Read the model definition and answer for the solid it produces. Units are mm, in the model's axes. A direction names the side the tool comes from. Coordinates: 2 decimals unless noted, no trailing zeros. Order: outer loops, then holes, each group sorted by start corner. A loop starts at its lowest first (then second) coordinate and runs counter-clockwise, first axis right, second up. Notation, with made-up numbers: (43, 0) - (101, 0) arc R16 cw to (101, 28) - close; hole circle Ø6 at (-32.5, 65). An arc over 180 degrees is marked (long way). Use one line per item in the form item = value.
```python
from build123d import *

# Parameters (mm, degrees)
F1_DEPTH = 0.5
F2_R     = 2.047791
F3_DEPTH = 9.5


with BuildPart() as f1:
    # F0 (on Top) → F1 (new body)
    with BuildSketch(Plane.XY):
        Polygon((16.35, 29.214), (-16.35, 29.214), (-16.35, 23.9715), (-9.35, 23.9715), (-9.35, 10.9715), (-16.35, 10.9715), (-16.35, 0), (-16.35, -10.9715), (-9.35, -10.9715), (-9.35, -23.9715), (-16.35, -23.9715), (-16.35, -29.214), (16.35, -29.214), (16.35, -23.9715), (9.35, -23.9715), (9.35, -10.9715), (16.35, -10.9715), (16.35, 0), (16.35, 10.9715), (9.35, 10.9715), (9.35, 23.9715), (16.35, 23.9715), align=None)
    extrude(amount=F1_DEPTH)

    # F2 (on Right) → F3 (join, symmetric)
    with BuildSketch(Plane.YZ):
        with BuildLine():
            Line((23.961247, 0), (10.961247, 0))
            ThreePointArc((10.961247, 0), (17.461247, -5.333223), (23.961247, 0))
        make_face()
        with Locations((17.461247, -2.643129)):
            Circle(F2_R, mode=Mode.SUBTRACT)
        with BuildLine():
            ThreePointArc((-23.961247, 0), (-17.461247, -5.333223), (-10.961247, 0))
            Line((-10.961247, 0), (-23.961247, 0))
        make_face()
        with Locations((-17.461247, -2.643129)):
            Circle(F2_R, mode=Mode.SUBTRACT)
    extrude(amount=F3_DEPTH, both=True)


solid = f1.part
```
(1) Which of the six approach directions +Z, -Z, +X, -X, +Y, -Y give full straight-line access (tool end or side, diameter ignored) to faces 3 (the flat face through (0, 27, 0)), 4 (the flat face through (0, 0, 0)), 5 (the cylindrical face through (-0.133, 15.836, -3.889)), 6 (the flat face through (0, -27, 0))?
Answer list:
face_3 = -Z, +X, -X, +Y
face_4 = -Z, +X, -X
face_5 = +X, -X
face_6 = -Z, +X, -X, -Y
(2) Straight lines are drawn through the part: L1, parallel to Y at x = 1, z = -0.05; L2, parallel to Y at x = -4.5, z = -1.05; L3, parallel to Y at x = -9, z = -3.2. For each, find the intervals that lie inside material, in ascending order.
Answer list:
L1 = -23.95 to -10.97, 10.97 to 23.95
L2 = -23.66 to -18.75, -16.17 to -11.26, 11.26 to 16.17, 18.75 to 23.66
L3 = -22.33 to -19.43, -15.49 to -12.59, 12.59 to 15.49, 19.43 to 22.33
(3) Section B-B, the plane z = -3.85 is taken. Write down the section's boundary in (x, y).
Answer list:
outline = (-9.5, -21.64) - (9.5, -21.64) - (9.5, -19.12) - (-9.5, -19.12) - close; (-9.5, -15.81) - (9.5, -15.81) - (9.5, -13.28) - (-9.5, -13.28) - close; (-9.5, 13.28) - (9.5, 13.28) - (9.5, 15.81) - (-9.5, 15.81) - close; (-9.5, 19.12) - (9.5, 19.12) - (9.5, 21.64) - (-9.5, 21.64) - close
(4) Section A-A, the plane x = -14 is taken. Write down the section's boundary in (y, z), then the cut area to 3 significant figures.
Answer list:
outline = (-29.21, 0) - (-23.97, 0) - (-23.97, 0.5) - (-29.21, 0.5) - close; (-10.97, 0) - (10.97, 0) - (10.97, 0.5) - (-10.97, 0.5) - close; (23.97, 0) - (29.21, 0) - (29.21, 0.5) - (23.97, 0.5) - close
area = 16.2 mm2
(5) Section C-C, the plane y = -18.5 is taken. Write down the section's boundary in (x, z), then the cut area to 3 significant figures.
Answer list:
outline = (-9.5, -5.25) - (9.5, -5.25) - (9.5, -4.41) - (-9.5, -4.41) - close; (-9.5, -0.88) - (9.5, -0.88) - (9.5, 0) - (9.35, 0) - (9.35, 0.5) - (-9.35, 0.5) - (-9.35, 0) - (-9.5, 0) - close
area = 42.1 mm2
(6) Section D-D, the plane x = 8.5 is taken. Write down the section's boundary in (y, z).
Answer list:
outline = (-29.21, 0) - (-23.96, 0) arc R6.63 ccw to (-10.96, 0) - (10.96, 0) arc R6.63 ccw to (23.96, 0) - (29.21, 0) - (29.21, 0.5) - (-29.21, 0.5) - close; hole circle Ø4.1 at (-17.46, -2.64); hole circle Ø4.1 at (17.46, -2.64)
(7) Given pin 1 Ø4 at (x, y) = (-5, 1) entering from -Z; pin 2 Ø1.6 at (y, z) = (16, -1.5) entering from +X; pin 3 Ø2 at (x, z) = (7, -1.5) entering from -Y, each flat-ended and moving along its own axis, determine where each tip first touches the part or whether it passes through.
Answer list:
pin_1 = 0
pin_2 = 9.5
pin_3 = -23.84
(8) The mould has two halves that part along Y. Classify faces 1 (the cylindrical face through (0.13, -17.59, -5.33)), 2 (the flat face through (-9.5, -16, -1)): +Y half, -Y half, draft (parallel to the pull), parting line (faces both ways), or undercut.
Answer list:
face_1 = undercut
face_2 = draft
